```python
from build123d import *

# Parameters (mm, degrees)
CROQUIS1_R              = 6.35
SALIENTE_EXTRUIR1_DEPTH = 12
CROQUIS2_R              = 4
SALIENTE_EXTRUIR2_DEPTH = 20
CROQUIS3_R              = 2.5
CORTAR_EXTRUIR1_DEPTH   = 10
CROQUIS4_R              = 2
CORTAR_EXTRUIR2_DEPTH   = 34.236200144
CROQUIS5_R              = 2
CORTAR_EXTRUIR3_DEPTH   = 34.236200182
CHAFL_N1_SIZE           = 0.8


with BuildPart() as part:
    # Croquis1 → Saliente-Extruir1 (new body)
    with BuildSketch(Plane.XY):
        Circle(CROQUIS1_R)
    extrude(amount=SALIENTE_EXTRUIR1_DEPTH)

    # Croquis2 → Saliente-Extruir2 (add)
    with BuildSketch(Plane.XY.offset(12)):
        Circle(CROQUIS2_R)
    extrude(amount=SALIENTE_EXTRUIR2_DEPTH)

    # Croquis3 → Cortar-Extruir1 (cut)
    with BuildSketch(Plane(origin=(0, 0, 0), x_dir=(-1, 0, 0), z_dir=(0, 0, -1))):
        Circle(CROQUIS3_R)
    extrude(amount=-CORTAR_EXTRUIR1_DEPTH, mode=Mode.SUBTRACT)

    # Croquis4 → Cortar-Extruir2 (cut, through all)
    with BuildSketch(Plane(origin=(0, 0, 0), x_dir=(0, 0, -1), z_dir=(1, 0, 0))):
        with Locations((-6, 0)):
            Circle(CROQUIS4_R)
    extrude(amount=-CORTAR_EXTRUIR2_DEPTH, mode=Mode.SUBTRACT)

    # Croquis5 → Cortar-Extruir3 (cut, through all)
    with BuildSketch(Plane(origin=(0, 0, 0), x_dir=(1, 0, 0), z_dir=(0, 1, 0))):
        with Locations(Location((0, -6, 0), (0, 0, 270))):
            Circle(CROQUIS5_R)
    extrude(amount=-CORTAR_EXTRUIR3_DEPTH, mode=Mode.SUBTRACT)

    # Chaflán1
    chafl_n1_edges = [part.edges().sort_by_distance(p)[0] for p in [
        (-6.35, 0, 0),
        (-6.35, 0, 12),
        (-4, 0, 32),
    ]]
    chamfer(chafl_n1_edges, length=CHAFL_N1_SIZE)


solid = part.part
```
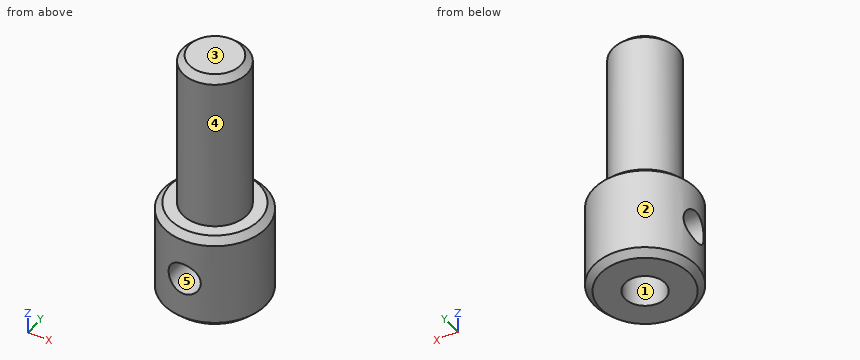
Check sheet for the modelled part. Datum: model origin and axes. Units: mm. Face numbers are marked on the shaded views. A direction names the side the tool comes from. Round coordinates to 2 decimals unless told otherwise and drop trailing zeros. Order: outer loops, then holes, each group sorted by start corner. A loop starts at its lowest first (then second) coordinate and runs counter-clockwise, first axis right, second up. Notation, with made-up numbers: (-21.75, 87.25) - (-14.75, 87.25) arc R29 cw to (-14.75, 122.25) - close; hole circle Ø7 at (-23.5, -33). An arc over 180 degrees is marked (long way). Answer as CSV lines item,"result". Start each with the question number.
1) Section check A-A (x = 0). Record the cut outline in (y, z), then the cut area to 3 significant figures.
2) Depth check by flat-ended pin: pin 1 (3 mm diameter, centred on x = 0, y = 0, fed in from -Z); pin 2 (3.5 mm diameter, centred on x = 0, z = 6, fed in from -Y); pin 3 (1.5 mm diameter, centred on x = 3.5, y = -2.5, fed in from +Z). Enter the tip coordinate at first touch or a pass-through.
3) Section check C-C (z = 5.5). Record the cut outline in (x, y), then the cut area to 3 significant figures.
4) Tool access check on the marked faces 1 and 2. Record the directions out of +Z, -Z, +X, -X, +Y, -Y that give a thin tool (end or side, any length) a straight path to the whole face; none if there is none.
5) Scan lines: probe 1 along Y at (x, z) = (0, 3); probe 2 along Z at (x, y) = (0.75, 0.5); probe 3 along Z at (x, y) = (-0.25, -3.5). Record each from-to range of solid material in increasing order.
6) Draft check along Z on the marked faces 3, 4 and 5. Enter one of: +Z half, -Z half, draft (parallel to the pull), parting line (faces both ways), or undercut.
7) Section check D-D (z = 17.5). Record the cut outline in (x, y), then the cut area to 3 significant figures.
Determined:
1,outline,"(-6.35, 0.8) - (-5.55, 0) - (-2.5, 0) - (-2.5, 4) - (-6.35, 4) - close; (-6.35, 8) - (-2.5, 8) - (-2.5, 10) - (2.5, 10) - (2.5, 0) - (5.55, 0) - (6.35, 0.8) - (6.35, 11.2) - (5.55, 12) - (4, 12) - (4, 31.2) - (3.2, 32) - (-3.2, 32) - (-4, 31.2) - (-4, 12) - (-5.55, 12) - (-6.35, 11.2) - close"
1,area,"245 mm^2"
2,pin 1,"z = 10"
2,pin 2,"y = 1.79"
2,pin 3,"z = 31.65"
3,outline,"(-6.05, -1.94) arc R6.35 ccw to (-1.94, -6.05) - (-1.94, -1.94) - close; (-6.05, 1.94) - (-1.58, 1.94) arc R2.5 cw to (1.94, -1.58) - (1.94, -6.05) arc R6.35 ccw (long way) to start"
3,area,"75.9 mm^2"
4,face 1,"-Z"
4,face 2,"+Z, -Z"
5,probe 1,"-6.35 to -2.5, 2.5 to 6.35"
5,probe 2,"10 to 32"
5,probe 3,"0 to 4.02, 7.98 to 31.69"
6,face 3,"+Z half"
6,face 4,"draft"
6,face 5,"undercut"
7,outline,"circle Ø8 at (0, 0)"
7,area,"50.3 mm^2"
